Could you check a few things on this model? Use its own coordinates, in mm. A direction names the side the tool comes from. Coordinates: 2 decimals unless noted, no trailing zeros. Write each loop counter-clockwise with the first axis right and the second up, starting at its lowest first coordinate (ties: lowest second). Pieces come first, ordered by that corner, then holes. Notation, with made-up numbers: (21, 81) - (78, 81) arc R26 ccw to (78, 101) - close; hole circle Ø4 at (78.25, 74). An arc over 180 degrees is marked (long way). Answer as a JSON object with one key per item and string values. Group by question number.
1) Please list where these lines run through material, in increasing order: line 1 along Y through (x, z) = (3, 51); line 2 along Z through (x, y) = (-13.5, 16.5); line 3 along Z through (x, y) = (-3.5, -6.5).
2) If we section it at C-C (x = 11): Write out the boundary of the cut face in (y, z), plus the area to 3 significant figures.
3) Will these pins go through, and if not, where does the flat tip stop? pin 1 Ø0.9 at (x, y) = (-18, 17.5) entering from +Z; pin 2 Ø3.5 at (x, y) = (13.5, 18) entering from +Z; pin 3 Ø18 at (x, z) = (3, 35.5) entering from +Y.
4) On a 3-axis mill with a long thin cutter (end or side, diameter ignored), from which of +Z, -Z, +X, -X, +Y, -Y can I reach the whole of each face in a straight line? I mean faces 1 (the flat face through (14, 18, 6)), 2 (the flat face through (16, 21, 48)), 3 (the flat face through (-20, 21, 6)), 4 (the flat face through (13, 18, 48)). Say none if no direction works.
5) If we section it at B-B (z = 9.5): Write out the boundary of the cut face in (x, y), plus the area to 3 significant figures.
6) If we section it at D-D (y = -10): Write out the boundary of the cut face in (x, z).
7) We'd pull the mould along Y, two halves only. Please class faces 5 (the flat face through (-20, 21, 48)), 6 (the flat face through (-19.679, -15.347, 26.706)), 7 (the cylindrical face through (-19.01, -13.21, 2.96)), 8 (the cylindrical face through (-19.01, -13.21, 50.96)): released by +Y, released by -Y, zero draft, split by the parting line, or undercut.
8) If we section it at A-A (z = 52): Write out the boundary of the cut face in (x, y).
```python
from build123d import *

# Parameters (mm, degrees)
SKETCH_1_W          = 42.3
SKETCH_1_H          = 42.3
SKETCH_1_R          = 1.5
EXTRUDE_1_DEPTH     = 6
EXTRUDE_2_DEPTH     = 42
SKETCH_3_W          = 42.3
SKETCH_3_H          = 42.3
EXTRUDE_3_DEPTH     = 6
SKETCH_4_R          = 2.5
EXTRUDE_4_DEPTH     = 24
SKETCH_4_3_R        = 11
SKETCH_4_3_R_2      = 2.5
EXTRUDE_5_DEPTH     = 2
CHAMFER_1_SIZE      = 3
CUT_EXTRUDE_START   = -6
SKETCH_5_R          = 1.5
CUT_EXTRUDE_1_DEPTH = 6
SKETCH_6_W          = 5.398834963
SKETCH_6_H          = 2.5
EXTRUDE_6_DEPTH     = 0.5
CHAMFER_2_SIZE      = 2


with BuildPart() as part:
    # 草图1 → 凸台-拉伸1 (new body)
    with BuildSketch(Plane.XY):
        with Locations((-2.012033722, 2.221867738)):
            Rectangle(SKETCH_1_W, SKETCH_1_H)
        with Locations((-17.512033722, 17.721867738)):
            Circle(SKETCH_1_R, mode=Mode.SUBTRACT)
        with Locations((13.487966278, 17.721867738)):
            Circle(SKETCH_1_R, mode=Mode.SUBTRACT)
        with Locations((-17.512033722, -13.278132262)):
            Circle(SKETCH_1_R, mode=Mode.SUBTRACT)
        with Locations((13.487966278, -13.278132262)):
            Circle(SKETCH_1_R, mode=Mode.SUBTRACT)
    extrude(amount=EXTRUDE_1_DEPTH)

    # 草图2 → 凸台-拉伸2 (add)
    with BuildSketch(Plane.XY.offset(6)):
        Polygon((-16.804926941, -18.221025481), (-22.454926941, -12.571025481), (-23.162033722, -11.8639187), (-23.162033722, 16.307654175), (-22.454926941, 17.014760956), (-16.804926941, 22.664760956), (-16.09782016, 23.371867738), (12.073752715, 23.371867738), (12.780859496, 22.664760956), (18.430859496, 17.014760956), (19.137966278, 16.307654175), (19.137966278, -11.8639187), (18.430859496, -12.571025481), (12.780859496, -18.221025481), (12.073752715, -18.928132262), (-16.09782016, -18.928132262), align=None)
    extrude(amount=EXTRUDE_2_DEPTH)

    # 草图3 → 凸台-拉伸3 (add)
    with BuildSketch(Plane.XY.offset(48)):
        with Locations((-2.012033722, 2.221867738)):
            Rectangle(SKETCH_3_W, SKETCH_3_H)
    extrude(amount=EXTRUDE_3_DEPTH)

    # 草图4 → 凸台-拉伸4 (add)
    with BuildSketch(Plane.XY.offset(54)):
        with Locations((-2.012033722, 2.221867738)):
            Circle(SKETCH_4_R)
    extrude(amount=EXTRUDE_4_DEPTH)

    # 草图4<3> → 凸台-拉伸5 (add)
    with BuildSketch(Plane.XY.offset(54)):
        with Locations((-2.012033722, 2.221867738)):
            Circle(SKETCH_4_3_R)
        with Locations((-2.012033722, 2.221867738)):
            Circle(SKETCH_4_3_R_2, mode=Mode.SUBTRACT)
    extrude(amount=EXTRUDE_5_DEPTH)

    # 倒角1
    chamfer_1_edges = [part.edges().sort_by_distance(p)[0] for p in [
        (-23.162033722, -18.928132262, 51),
        (-23.162033722, -18.928132262, 3),
        (19.137966278, -18.928132262, 51),
        (19.137966278, -18.928132262, 3),
        (19.137966278, 23.371867738, 51),
        (19.137966278, 23.371867738, 3),
        (-23.162033722, 23.371867738, 51),
        (-23.162033722, 23.371867738, 3),
    ]]
    chamfer(chamfer_1_edges, length=CHAMFER_1_SIZE)

    # 草图5 → 切除-拉伸1 (cut)
    with BuildSketch(Plane.XY.offset(54).offset(CUT_EXTRUDE_START)):
        with Locations((-17.512033722, 17.721867738)):
            Circle(SKETCH_5_R)
        with Locations((13.487966278, 17.721867738)):
            Circle(SKETCH_5_R)
        with Locations((13.487966278, -13.278132262)):
            Circle(SKETCH_5_R)
        with Locations((-17.512033722, -13.278132262)):
            Circle(SKETCH_5_R)
    extrude(amount=CUT_EXTRUDE_1_DEPTH, mode=Mode.SUBTRACT)

    # 草图6 → 凸台-拉伸6 (add)
    with BuildSketch(Plane(origin=(0, 23.371867738, 0), x_dir=(1, 0, 0), z_dir=(0, 1, 0))):
        with Locations((-2.012033723, -7.25)):
            Rectangle(SKETCH_6_W, SKETCH_6_H)
    extrude(amount=EXTRUDE_6_DEPTH)

    # 倒角2
    chamfer_2_edges = [part.edges().sort_by_distance(p)[0] for p in [
        (-13.012033722, 2.221867738, 56),
    ]]
    chamfer(chamfer_2_edges, length=CHAMFER_2_SIZE - 0.0001)  # a hair under: the kernel refuses the full size


solid = part.part
```
Here are the results:
{
 "1": {"line 1": "y = -18.93 to 23.37", "line 2": "z = 0 to 54", "line 3": "z = 0 to 56"},
 "2": {"outline": "(-18.93, 0) - (23.37, 0) - (23.37, 54) - (-18.93, 54) - close", "area": "2,280 mm²"},
 "3": {"pin 1": "stops at z = 48", "pin 2": "stops at z = 54", "pin 3": "stops at y = 23.37"},
 "4": {"face 1": "-Z", "face 2": "+X, +Y", "face 3": "-X, +Y", "face 4": "+Z"},
 "5": {"outline": "(-23.16, -11.86) - (-16.1, -18.93) - (12.07, -18.93) - (19.14, -11.86) - (19.14, 16.31) - (12.07, 23.37) - (-16.1, 23.37) - (-23.16, 16.31) - close", "area": "1,690 mm²"},
 "6": {"outline": "(-23.16, 0) - (19.14, 0) - (19.14, 54) - (-23.16, 54) - close"},
 "7": {"face 5": "zero draft", "face 6": "released by -Y", "face 7": "undercut", "face 8": "undercut"},
 "8": {"outline": "(-23.16, -15.93) - (-20.16, -18.93) - (16.14, -18.93) - (19.14, -15.93) - (19.14, 20.37) - (16.14, 23.37) - (-20.16, 23.37) - (-23.16, 20.37) - close; hole circle Ø3 at (-17.51, -13.28); hole circle Ø3 at (-17.51, 17.72); hole circle Ø3 at (13.49, -13.28); hole circle Ø3 at (13.49, 17.72)"}
}
